Autodesk Inventor part; units mm, degrees
ref_plane "YZ Plane" through (0, 0, 0) normal (1, 0, 0) x (0, 1, 0)
ref_plane "XZ Plane" through (0, 0, 0) normal (0, 1, 0) x (-1, 0, 0)
ref_plane "XY Plane" through (0, 0, 0) normal (0, 0, 1) x (1, 0, 0)
sketch "Sketch1" plane through (0, 0, 0) normal (1, 0, 0) x (0, 1, 0)
  line L0 (-0.825, 1) -> (0.825, 1)
  line L1 (0.825, -1) -> (-0.825, -1)
  line L2 (-0.825, -1) -> (-0.825, 1) construction
  line L3 (-0.825, 1) -> (0.825, -1) construction
  line L4 (0.825, 1) -> (-0.825, -1) construction
  arc A0 (0.825, 1) -> (0.825, -1) centre (0.825, 0) ccw
  line L5 (-0.825, 1) -> (-1.275, 0)
  line L6 (-1.275, 0) -> (-0.825, -1)
  point P0 (0, 0)
  dimension "d0" = 2
  dimension "d1" = 1.65
  dimension "d9" = 2.1
extrude "Extrusion1" add sketch "Sketch1" along normal mid plane 11
fillet "Fillet1" radius 0.05 2 edges at (0, 0.825, 1) (0, 0.825, -1)
fillet "Fillet1" radius 0.15 3 edges at (0, -0.825, -1) (0, -0.825, 1) (0, -1.275, 0)
sketch "Sketch2" plane through (0, 0, 0) normal (1, 0, 0) x (0, 1, 0)
  arc A0 (0.825, 1) -> (0.825, -1) centre (0.825, 0) ccw
  circle A1 centre (0.825, 0) radius 1
  line L0 (-0.728, 1) -> (0.3778, 1)
  line L1 (0.3778, 1) -> (0.825, 1)
  line L2 (0.825, 1) -> (0.825, -1)
  line L3 (-0.728, -1) -> (0.3778, -1)
  line L4 (0.825, -1) -> (0.3778, -1)
  arc A2 (-1.2473, 0.0616) -> (-1.2473, -0.0616) centre (-1.1105, 0) ccw
  line L5 (-1.2473, -0.0616) -> (-0.8648, -0.9116)
  arc A3 (-0.8648, -0.9116) -> (-0.728, -1) centre (-0.728, -0.85) ccw
  line L6 (-0.728, -1) -> (0.3778, -1)
  arc A4 (0.3778, -1) -> (0.3991, -0.9048) centre (0.3778, -0.95) ccw
  arc A5 (0.3991, 0.9048) -> (0.3991, -0.9048) centre (0.825, 0) ccw
  arc A6 (0.3991, 0.9048) -> (0.3778, 1) centre (0.3778, 0.95) ccw
  line L7 (0.3778, 1) -> (-0.728, 1)
  arc A7 (-0.728, 1) -> (-0.8648, 0.9116) centre (-0.728, 0.85) ccw
  line L8 (-0.8648, 0.9116) -> (-1.2473, 0.0616)
  point P0 (0, 0)
  point P1 (0.825, 1)
  point P2 (0.3991, 0.9048)
  point P3 (0.3991, -0.9048)
  point P4 (0.3778, -1)
extrude "graphite" add sketch "Sketch2" along normal mid plane 11 contours L2 A0 | A0 A6 L1 | A1 L2 | L4 A4 A0
properties part number "ApexSeal"
Here's how the part is built. I have some questions about the finished solid (model axes, mm). Coordinates: 2 decimals unless noted, no trailing zeros. Order: outer loops, then holes, each group sorted by start corner. A loop starts at its lowest first (then second) coordinate and runs counter-clockwise, first axis right, second up.
Item 1: I need wall thicknesses on probe 1 along Y at (x, z) = (-3.75, -0.35); probe 2 along Y at (x, z) = (-2.5, 0.9); probe 3 along Z at (x, y) = (2.25, 1.35). Which ranges of each line are inside material? Lowest first, please.
Response values:
probe 1: y = -1.12 to 1.76
probe 2: y = -0.87 to 1.26
probe 3: z = -0.85 to 0.85
Item 2: If we section it at C-C, the plane y = 1.1: List the corners of the cut face in (x, z) for me, then the cut area to 3 significant figures.
Response values:
outline: (-5.5, -0.96) - (5.5, -0.96) - (5.5, 0.96) - (-5.5, 0.96) - close
area: 21.2 mm2
Item 3: If we section it at B-B, the plane z = -0.55: List the corners of the cut face in (x, y) for me.
Response values:
outline: (-5.5, -1.03) - (5.5, -1.03) - (5.5, 1.66) - (-5.5, 1.66) - close
